```python
from build123d import *

# Parameters (mm, degrees)
SALIENTE_EXTRUIR1_DEPTH = 10
CROQUIS2_R              = 7.5
SALIENTE_EXTRUIR2_DEPTH = 2
CROQUIS3_R              = 3.75
CROQUIS3_R_2            = 0.75
CORTAR_EXTRUIR1_DEPTH   = 6.5
CROQUIS4_W              = 1
CROQUIS4_H              = 5
CROQUIS4_W_2            = 5
CROQUIS4_H_2            = 1
SALIENTE_EXTRUIR3_DEPTH = 7.5
CORTAR_EXTRUIR2_REACH   = 20.554
CROQUIS5_R              = 1.25
CROQUIS6_R              = 1.25
CORTAR_EXTRUIR3_DEPTH   = 1
REDONDEO1_R             = 2


with BuildPart() as part:
    # Croquis1 → Saliente-Extruir1 (new body)
    with BuildSketch(Plane(origin=(0, 0, 0), x_dir=(1, 0, 0), z_dir=(0, 1, 0))):
        with BuildLine():
            Line((6, 2.5), (6, -2.5))
            ThreePointArc((6, -2.5), (0, -6.5), (-6, -2.5))
            Line((-6, -2.5), (-6, 2.5))
            ThreePointArc((-6, 2.5), (0, 6.5), (6, 2.5))
        make_face()
    extrude(amount=SALIENTE_EXTRUIR1_DEPTH)

    # Croquis2 → Saliente-Extruir2 (add)
    with BuildSketch(Plane(origin=(0, 10, 0), x_dir=(1, 0, 0), z_dir=(0, 1, 0))):
        with Locations(Location((0, 0, 0), (0, 0, 270))):
            Circle(CROQUIS2_R)
    extrude(amount=SALIENTE_EXTRUIR2_DEPTH)

    # Croquis3 → Cortar-Extruir1 (cut)
    with BuildSketch(Plane(origin=(0, 12, 0), x_dir=(1, 0, 0), z_dir=(0, 1, 0))):
        with Locations(Location((0, 0, 0), (0, 0, 270))):
            Circle(CROQUIS3_R)
        with Locations(Location((0, 0, 0), (0, 0, 270))):
            Circle(CROQUIS3_R_2, mode=Mode.SUBTRACT)
    extrude(amount=-CORTAR_EXTRUIR1_DEPTH, mode=Mode.SUBTRACT)

    # Croquis4 → Saliente-Extruir3 (add)
    with BuildSketch(Plane.XZ):
        with Locations((-4, 0)):
            Rectangle(CROQUIS4_W, CROQUIS4_H)
        with Locations((4, 0)):
            Rectangle(CROQUIS4_W, CROQUIS4_H)
        with Locations((0, 4)):
            Rectangle(CROQUIS4_W_2, CROQUIS4_H_2)
    extrude(amount=SALIENTE_EXTRUIR3_DEPTH)

    # Cortar-Extruir2: up to this face of the body (flat: up to its plane)
    cortar_extruir2_end = Plane(part.part.faces().sort_by_distance((4.5, -3.75, 0))[0])
    # Croquis5 → Cortar-Extruir2 (cut, up to the picked face)
    with BuildSketch(Plane.ZY.offset(4.5), mode=Mode.PRIVATE) as cortar_extruir2_sk1:
        with Locations((0, -4.997728335)):
            Circle(CROQUIS5_R)
    cortar_extruir2_tool1 = split(extrude(cortar_extruir2_sk1.sketch, amount=-CORTAR_EXTRUIR2_REACH, mode=Mode.PRIVATE), bisect_by=cortar_extruir2_end, keep=Keep.BOTH, mode=Mode.PRIVATE)
    add(cortar_extruir2_tool1.solids().sort_by(Axis((-4.5, -4.997728, 0), (1, 0, 0)))[0], mode=Mode.SUBTRACT)

    # Croquis6 → Cortar-Extruir3 (cut)
    with BuildSketch(Plane.XY.offset(4.5)):
        with Locations((0, -5)):
            Circle(CROQUIS6_R)
    extrude(amount=-CORTAR_EXTRUIR3_DEPTH, mode=Mode.SUBTRACT)

    # Redondeo1
    redondeo1_edges = [part.edges().sort_by_distance(p)[0] for p in [
        (-4, -7.5, 2.5),
        (-4, -7.5, -2.5),
        (4, -7.5, 2.5),
        (4, -7.5, -2.5),
        (2.5, -7.5, 4),
        (-2.5, -7.5, 4),
    ]]
    fillet(redondeo1_edges, radius=REDONDEO1_R)


solid = part.part
```
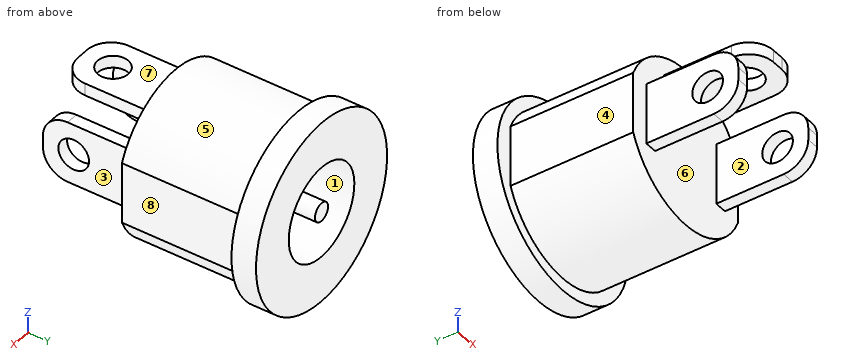
Build history of the part. All positions in model axes, mm. Face numbers are marked on the shaded views. A direction names the side the tool comes from. Coordinates: 2 decimals unless noted, no trailing zeros. Order: outer loops, then holes, each group sorted by start corner. A loop starts at its lowest first (then second) coordinate and runs counter-clockwise, first axis right, second up.
Item 1: Tool access for the marked faces 1, 2, 3 and 4: list every direction of +Z, -Z, +X, -X, +Y, -Y with a clear straight run to the whole face (end or side of a thin tool).
Filled in:
face 1: +Y
face 2: +Z, -Z, -Y
face 3: +Z, -Z, +X, -Y
face 4: +Z, -Z, -X, -Y
Item 2: Saw through at D-D on y = 5.25. List the corners of the cut face in (x, z), then the cut area to 3 significant figures.
Filled in:
outline: (-6, -2.5) arc R6.5 ccw to (6, -2.5) - (6, 2.5) arc R6.5 ccw to (-6, 2.5) - close
area: 129 mm2
Item 3: Saw through at C-C on y = -4.5. List the corners of the cut face in (x, z).
Filled in:
outline: (-4.5, -2.5) - (-3.5, -2.5) - (-3.5, -1.15) - (-4.5, -1.15) - close; (-4.5, 1.15) - (-3.5, 1.15) - (-3.5, 2.5) - (-4.5, 2.5) - close; (-2.5, 3.5) - (-1.15, 3.5) - (-1.15, 4.5) - (-2.5, 4.5) - close; (1.15, 3.5) - (2.5, 3.5) - (2.5, 4.5) - (1.15, 4.5) - close; (3.5, -2.5) - (4.5, -2.5) - (4.5, -1.15) - (3.5, -1.15) - close; (3.5, 1.15) - (4.5, 1.15) - (4.5, 2.5) - (3.5, 2.5) - close
Item 4: Saw through at B-B on x = 0.25. List the corners of the cut face in (y, z), then the cut area to 3 significant figures.
Filled in:
outline: (-7.5, 3.5) - (-6.22, 3.5) - (-6.22, 4.5) - (-7.5, 4.5) - close; (-3.78, 3.5) - (0, 3.5) - (0, -6.5) - (10, -6.5) - (10, -7.5) - (12, -7.5) - (12, -3.74) - (5.5, -3.74) - (5.5, -0.71) - (12, -0.71) - (12, 0.71) - (5.5, 0.71) - (5.5, 3.74) - (12, 3.74) - (12, 7.5) - (10, 7.5) - (10, 6.5) - (0, 6.5) - (0, 4.5) - (-3.78, 4.5) - close
area: 125 mm2
Item 5: Drill centre lines: L1, parallel to X at y = 8, z = 0; L2, parallel to Y at x = 4.25, z = 0; L3, parallel to Y at x = -3.65, z = 0. Where is each one in solid material? Low to high.
Filled in:
L1: x = -6 to -3.75, -0.75 to 0.75, 3.75 to 6
L2: y = -7.5 to -6.25, -3.75 to 12
L3: y = -7.5 to -6.25, -3.75 to 5.5
Item 6: Mould opens along X. For the marked faces 5, 6, 7 and 8 say: released by +X, released by -X, zero draft, split by the parting line, or undercut.
Filled in:
face 5: split by the parting line
face 6: undercut
face 7: zero draft
face 8: released by +X
Item 7: Saw through at A-A on z = 0. State how many separate pieces and enclosed holes the cut face has, then the cut area to 3 significant figures.
Filled in:
separate pieces: 3
enclosed holes: 0
area: 121 mm2
Item 8: Drop flat-ended pins along their axis: pin 1 Ø2.5 at (y, z) = (-4, -1) entering from -X; pin 2 Ø3 at (x, z) = (-1, -5.5) entering from -Y; pin 3 Ø4 at (y, z) = (-5, 0) entering from +X; pin 4 Ø2 at (x, y) = (0, -5) entering from -Z. Give the stop position or say it passes through.
Filled in:
pin 1: stops at x = -4.5
pin 2: stops at y = 0
pin 3: stops at x = 4.5
pin 4: passes through
